from build123d import *

# Parameters (mm, degrees)
SKETCH1_R           = 4
BOSS_EXTRUDE1_DEPTH = 18
SKETCH3_R           = 13.976554855
SKETCH3_R_2         = 8.660254038
CUT_EXTRUDE1_DEPTH  = 3


with BuildPart() as part:
    # Sketch1 → Boss-Extrude1 (new body)
    with BuildSketch(Plane(origin=(0, 0, 0), x_dir=(1, 0, 0), z_dir=(0, 1, 0))):
        Polygon((10, 0), (5, 8.660254038), (-5, 8.660254038), (-10, 0), (-5, -8.660254038), (5, -8.660254038), align=None)
        with Locations(Location((2, 2, 0), (0, 0, 270))):
            Circle(SKETCH1_R, mode=Mode.SUBTRACT)
    extrude(amount=BOSS_EXTRUDE1_DEPTH)

    # Sketch3 → Cut-Extrude1 (cut)
    with BuildSketch(Plane(origin=(0, 18, 0), x_dir=(1, 0, 0), z_dir=(0, 1, 0))):
        Circle(SKETCH3_R)
        with Locations(Location((0, 0, 0), (0, 0, 270))):
            Circle(SKETCH3_R_2, mode=Mode.SUBTRACT)
    extrude(amount=-CUT_EXTRUDE1_DEPTH, mode=Mode.SUBTRACT)


solid = part.part
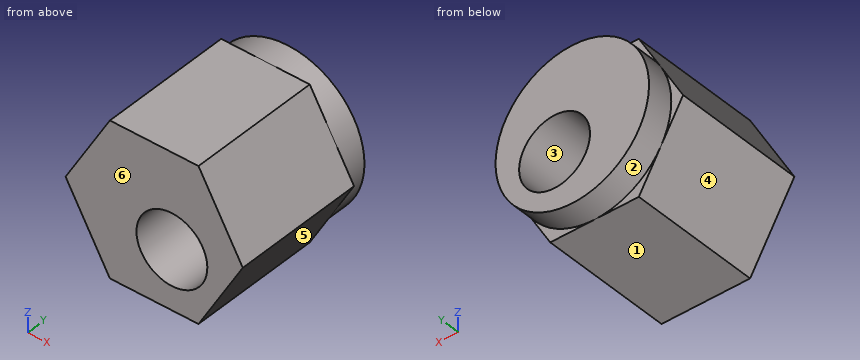
Source: CAD feature listing. Evaluate the final solid. Frame: model axes, mm. Face numbers are marked on the shaded views. A direction names the side the tool comes from. Round coordinates to 2 decimals unless told otherwise and drop trailing zeros. Loops run counter-clockwise (first coordinate to the right, second up) from the corner with the lowest first, then second, coordinate; pieces in that order, holes last. Notation, with made-up numbers: M 30.25,-14.75 L 69.25,-14.75 A11 ccw 69.25,2.25 Z; hole C 82,12 d3. An arc over 180 degrees is marked long. Return JSON: item names as keys, results as strings. Group by question number.
1. Material intervals for line 1 along X through (y, z) = (9.25, -1.5); line 2 along Z through (x, y) = (-1.25, 3.25); line 3 along X through (y, z) = (14.5, -5), sorted ascending. Write a range as from..to.
2. Section query A-A on y = 8. Output: boundary loops of the cut face in (x, z).
3. Pin query (flat end, axial travel): pin 1 (1 mm diameter, centred on x = 3.5, z = 0.5, fed in from +Y); pin 2 (2.5 mm diameter, centred on x = -9, z = 0.5, fed in from +Y); pin 3 (2 mm diameter, centred on y = 10.5, z = 6, fed in from -X); pin 4 (5 mm diameter, centred on y = 8, z = 5, fed in from -X). Return the tip coordinate at first contact, or that it passes through.
4. Reachability of the marked faces 1 and 2 from +Z, -Z, +X, -X, +Y, -Y: full face, straight path, thin tool, end or side. Return the list, or none.
5. Section query B-B on x = 2. Output: boundary loops of the cut face in (y, z), and give its area (3 significant figures).
6. Section query D-D on z = 6. Output: boundary loops of the cut face in (x, y) (3 decimals).
7. Mould query, pull axis X, two halves, no side actions, for the marked faces 3, 4, 5 and 6. Classes: released by +X, released by -X, zero draft, split by the parting line, or undercut.
8. Section query C-C on z = -0.5. Output: boundary loops of the cut face in (x, y).
Checks:
{
 "1": {"line 1": "x = -9.13..-1.97, 5.97..9.13", "line 2": "z = -8.66..-4.33, 0.33..8.66", "line 3": "x = -7.11..-0.65, 4.65..7.11"},
 "2": {"outline": "M -10,0 L -5,-8.66 L 5,-8.66 L 10,0 L 5,8.66 L -5,8.66 Z; hole C 2,-2 d8"},
 "3": {"pin 1": "passes through", "pin 2": "stops at y = 18", "pin 3": "stops at x = -7.11", "pin 4": "stops at x = -8.56"},
 "4": {"face 1": "-Z, +X, -X, +Y, -Y", "face 2": "+Y"},
 "5": {"outline": "M 0,-8.66 L 15,-8.66 L 15,-8.43 L 18,-8.43 L 18,-6 L 0,-6 Z; M 0,2 L 18,2 L 18,8.43 L 15,8.43 L 15,8.66 L 0,8.66 Z", "area": "166 mm²"},
 "6": {"outline": "M -6.536,0 L 6.536,0 L 6.536,15 L 6.245,15 L 6.245,18 L -6.245,18 L -6.245,15 L -6.536,15 Z"},
 "7": {"face 3": "undercut", "face 4": "released by -X", "face 5": "released by +X", "face 6": "zero draft"},
 "8": {"outline": "M -9.71,0 L -1.71,0 L -1.71,18 L -8.65,18 L -8.65,15 L -9.71,15 Z; M 5.71,0 L 9.71,0 L 9.71,15 L 8.65,15 L 8.65,18 L 5.71,18 Z"}
}
